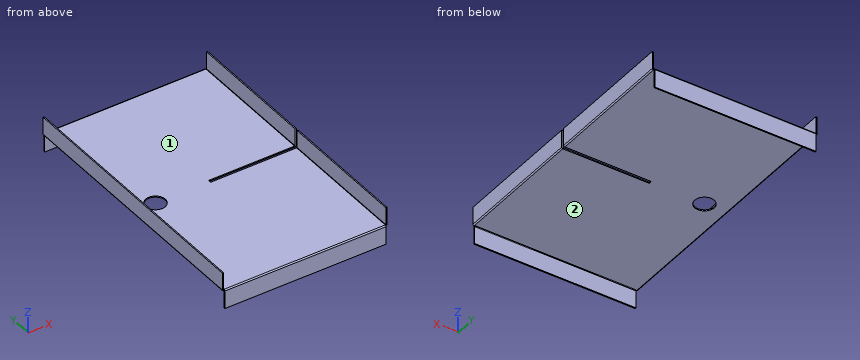
from build123d import *

# Parameters (mm, degrees)
F1_DEPTH      = 211.5
F1_DEPTH_BACK = 70
F3_DEPTH      = 347
F3_DEPTH_BACK = 347
F5_W          = 233.843906
F5_H          = 8
F6_DEPTH      = 80
F7_R          = 25.5
F8_DEPTH      = 12.5


with BuildPart() as f1:
    # F0 (on Right) → F1 (new body, two sides)
    with BuildSketch(Plane.YZ) as f1_sk:
        with BuildLine():
            ThreePointArc((-347, 4.5), (-349.12132, 3.62132), (-350, 1.5))
            Line((-350, 1.5), (-350, -45.5))
            Line((-350, -45.5), (-347, -45.5))
            Line((-347, -45.5), (-347, 0))
            ThreePointArc((-347, 0), (-346.56066, 1.06066), (-345.5, 1.5))
            Line((-345.5, 1.5), (345.5, 1.5))
            ThreePointArc((345.5, 1.5), (346.56066, 1.06066), (347, 0))
            Line((347, 0), (347, -45.5))
            Line((347, -45.5), (350, -45.5))
            Line((350, -45.5), (350, 1.5))
            ThreePointArc((350, 1.5), (349.12132, 3.62132), (347, 4.5))
            Line((347, 4.5), (-347, 4.5))
        make_face()
    extrude(amount=F1_DEPTH)
    extrude(f1_sk.sketch, amount=-F1_DEPTH_BACK)

    # F2 (on Front) → F3 (join, two sides)
    with BuildSketch(Plane.XZ) as f3_sk:
        with BuildLine():
            Line((216, 50), (213, 50))
            Line((213, 50), (213, 4.5))
            ThreePointArc((213, 4.5), (212.56066, 3.43934), (211.5, 3))
            Line((211.5, 3), (211.5, 1.5))
            Line((211.5, 1.5), (213, 1.5))
            ThreePointArc((213, 1.5), (215.12132, 2.37868), (216, 4.5))
            Line((216, 4.5), (216, 50))
        make_face()
    extrude(amount=F3_DEPTH)
    extrude(f3_sk.sketch, amount=-F3_DEPTH_BACK)

    # F4: F1 across plane


with BuildPart() as f1_1:
    add(f1.part)
    add(f1.part.mirror(Plane.YZ))

    # F5 (on Top) → F6 (cut)
    with BuildSketch(Plane.XY):
        with Locations((102.921953, 0)):
            Rectangle(F5_W, F5_H)
    extrude(amount=F6_DEPTH, mode=Mode.SUBTRACT)

    # F7 (on face) → F8 (cut, symmetric)
    with BuildSketch(Plane(origin=(0, 0, 1.5), x_dir=(1, 0, 0), z_dir=(0, 0, -1))):
        with Locations((-156, 0)):
            Circle(F7_R)
    extrude(amount=F8_DEPTH, both=True, mode=Mode.SUBTRACT)


solid = f1_1.part
The model under review builds one solid part; all positions refer to its coordinate system, in mm. Face numbers are marked on the shaded views. Round coordinates to 2 decimals unless told otherwise and drop trailing zeros. Loops run counter-clockwise (first coordinate to the right, second up) from the corner with the lowest first, then second, coordinate; pieces in that order, holes last. Notation, with made-up numbers: M 67.5,19 L 85.5,19 A27 cw 85.5,55 Z; hole C 42.5,20.25 d7. An arc over 180 degrees is marked long. Answer as CSV lines item,"result".
1. Insertion check: pin 1 Ø3.5 at (x, z) = (215, 23.5) entering from +Y; pin 2 Ø6 at (x, y) = (-86, 193) entering from +Z; pin 3 Ø1.5 at (y, z) = (109.5, 3.5) entering from +X. Each pin has a flat end and moves straight along its axis. Give the tip position at first contact, or say it passes through.
Outcome:
pin 1,"stops at y = 347"
pin 2,"stops at z = 4.5"
pin 3,"stops at x = 215.99"
2. We need section D-D (y = 281.5). Give the boundary of the cut face in (x, z), plus the area to 3 significant figures.
Outcome:
outline,"M -216,4.5 A3 ccw -213,1.5 L 213,1.5 A3 ccw 216,4.5 L 216,50 L 213,50 L 213,4.5 A1.5 cw 211.5,3 L 211.5,4.5 L -211.5,4.5 L -211.5,3 A1.5 cw -213,4.5 L -213,50 L -216,50 Z"
area,"1,560 mm2"
3. Draft analysis for pull direction Y (two halves, no side actions). For the marked faces 1 and 2, state which applies: pulls with the +Y half, pulls with the -Y half, needs draft (parallel to the pull), parting line crosses it, or undercut.
Outcome:
face 1,"needs draft"
face 2,"undercut"
4. We need section B-B (z = 32). Give the boundary of the cut face in (x, y), plus the area to 3 significant figures.
Outcome:
outline,"M -216,-347 L -213,-347 L -213,347 L -216,347 Z; M 213,-347 L 216,-347 L 216,-4 L 213,-4 Z; M 213,4 L 216,4 L 216,347 L 213,347 Z"
area,"4,140 mm2"
5. To check wall thickness, follow L1, parallel to X at y = -137.5, z = 33.5; L2, parallel to Y at x = -173, z = -10.5; L3, parallel to Y at x = -156, z = 2.25. State the ranges of each line that lie inside material, in increasing order. Write a range as [from, to].
Outcome:
L1,"x = [-216, -213], [213, 216]"
L2,"y = [-350, -347], [347, 350]"
L3,"y = [-349.9, -25.5], [25.5, 349.9]"
6. We need section A-A (x = 169). Give the boundary of the cut face in (y, z).
Outcome:
outline,"M -350,-45.5 L -347,-45.5 L -347,0 A1.5 cw -345.5,1.5 L -4,1.5 L -4,4.5 L -347,4.5 A3 ccw -350,1.5 Z; M 4,1.5 L 345.5,1.5 A1.5 cw 347,0 L 347,-45.5 L 350,-45.5 L 350,1.5 A3 ccw 347,4.5 L 4,4.5 Z"
7. We need section C-C (x = -91.5). Give the boundary of the cut face in (y, z).
Outcome:
outline,"M -350,-45.5 L -347,-45.5 L -347,0 A1.5 cw -345.5,1.5 L 345.5,1.5 A1.5 cw 347,0 L 347,-45.5 L 350,-45.5 L 350,1.5 A3 ccw 347,4.5 L -347,4.5 A3 ccw -350,1.5 Z"
